For this review, take the finished solid that the model builds, in its own axes (mm). A direction names the side the tool comes from. Round coordinates to 2 decimals unless told otherwise and drop trailing zeros. Write each loop counter-clockwise with the first axis right and the second up, starting at its lowest first coordinate (ties: lowest second). Pieces come first, ordered by that corner, then holes. Notation, with made-up numbers: (-27, 74) -> (13, 74) arc R29 ccw to (13, 100) -> close; hole circle Ø3 at (68, 24). An arc over 180 degrees is marked (long way). Answer in a Markdown table with one row per item. Add a question column.
```python
from build123d import *

# Parameters (mm, degrees)
SKETCH1_R           = 92.5
BOSS_EXTRUDE1_DEPTH = 5
SKETCH2_R           = 72
BOSS_EXTRUDE2_DEPTH = 5
SKETCH3_R           = 67
CUT_EXTRUDE1_DEPTH  = 11
SKETCH4_W           = 140
SKETCH4_H           = 70
BOSS_EXTRUDE3_DEPTH = 5
SKETCH6_W           = 60
SKETCH6_H           = 5
BOSS_EXTRUDE4_DEPTH = 20
FILLET1_R           = 2.5
SKETCH7_W           = 110
SKETCH7_H           = 25
BOSS_EXTRUDE5_DEPTH = 5
SKETCH11_R          = 2
CUT_EXTRUDE4_DEPTH  = 5
SKETCH12_R          = 2.5
CUT_EXTRUDE5_DEPTH  = 5
SKETCH13_R          = 2
CUT_EXTRUDE6_DEPTH  = 5


with BuildPart() as part:
    # Sketch1 → Boss-Extrude1 (new body)
    with BuildSketch(Plane.XY):
        Circle(SKETCH1_R)
    extrude(amount=BOSS_EXTRUDE1_DEPTH)

    # Sketch2 → Boss-Extrude2 (add)
    with BuildSketch(Plane.XY.offset(5)):
        Circle(SKETCH2_R)
    extrude(amount=BOSS_EXTRUDE2_DEPTH)

    # Sketch3 → Cut-Extrude1 (cut, through all)
    with BuildSketch(Plane(origin=(0, 0, 0), x_dir=(-1, 0, 0), z_dir=(0, 0, -1))):
        Circle(SKETCH3_R)
    extrude(amount=-CUT_EXTRUDE1_DEPTH, mode=Mode.SUBTRACT)

    # Sketch4 → Boss-Extrude3 (add)
    with BuildSketch(Plane(origin=(0, 0, 0), x_dir=(-1, 0, 0), z_dir=(0, 0, -1))):
        with Locations((0, -5)):
            Rectangle(SKETCH4_W, SKETCH4_H)
    extrude(amount=-BOSS_EXTRUDE3_DEPTH)

    # Sketch6 → Boss-Extrude4 (add)
    with BuildSketch(Plane.XY.offset(5)):
        with Locations((0, -37.5)):
            Rectangle(SKETCH6_W, SKETCH6_H)
    extrude(amount=BOSS_EXTRUDE4_DEPTH)

    # Fillet1
    fillet1_edges = [part.edges().sort_by_distance(p)[0] for p in [
        (0, -40, 0),
    ]]
    fillet(fillet1_edges, radius=FILLET1_R)

    # Sketch7 → Boss-Extrude5 (add)
    with BuildSketch(Plane(origin=(0, 0, 0), x_dir=(-1, 0, 0), z_dir=(0, 0, -1))):
        with Locations((0, -55)):
            Rectangle(SKETCH7_W, SKETCH7_H)
    extrude(amount=-BOSS_EXTRUDE5_DEPTH)

    # Sketch11 → Cut-Extrude4 (cut)
    with BuildSketch(Plane(origin=(0, 0, 0), x_dir=(-1, 0, 0), z_dir=(0, 0, -1))):
        with Locations((-30, -30)):
            Circle(SKETCH11_R)
        with Locations((-30, 20)):
            Circle(SKETCH11_R)
        with Locations((30, 20)):
            Circle(SKETCH11_R)
        with Locations((30, -30)):
            Circle(SKETCH11_R)
    extrude(amount=-CUT_EXTRUDE4_DEPTH, mode=Mode.SUBTRACT)

    # Sketch12 → Cut-Extrude5 (cut)
    with BuildSketch(Plane(origin=(0, 0, 0), x_dir=(-1, 0, 0), z_dir=(0, 0, -1))):
        with Locations((0, -78.5)):
            Circle(SKETCH12_R)
        with Locations((-78.5, 0)):
            Circle(SKETCH12_R)
        with Locations((0, 78.5)):
            Circle(SKETCH12_R)
        with Locations((78.5, 0)):
            Circle(SKETCH12_R)
    extrude(amount=-CUT_EXTRUDE5_DEPTH, mode=Mode.SUBTRACT)

    # Sketch13 → Cut-Extrude6 (cut)
    with BuildSketch(Plane(origin=(0, -35, 0), x_dir=(1, 0, 0), z_dir=(0, 1, 0))):
        with Locations((-20, -15)):
            Circle(SKETCH13_R)
        with Locations((20, -15)):
            Circle(SKETCH13_R)
    extrude(amount=-CUT_EXTRUDE6_DEPTH, mode=Mode.SUBTRACT)


solid = part.part
```
1. For L1, parallel to Z at x = 20, y = -37; L2, parallel to Y at x = -30, z = 3.7; L3, parallel to Y at x = 29.5, z = 1.5, list the stretches that pass through material, from the lowest coordinate up. Write a range as [from, to].
2. We need section A-A (z = 7.75). Write out the cut boundary in (x, y).
3. The part is to be moulded in two halves that separate along X. For faces 1 (the flat face through (0, -37, 25)), 2 (the cylindrical face through (29.077, -31.774, 2.465)), 3 (the cylindrical face through (49.727, 77.996, 2.465)), say which applies: pulls with the +X half, pulls with the -X half, needs draft (parallel to the pull), parting line crosses it, or undercut.
4. Tool access review of faces 4 (the flat face through (-1, 1, 0)), 5 (the flat face through (1, -40, 14)), 6 (the cylindrical face through (-9.373, 71.387, 7.465)): name each direction out of +Z, -Z, +X, -X, +Y, -Y from which nothing blocks a thin tool from reaching the whole face with its end or side.
5. We need section B-B (x = 0). Count the separate pieces of the cut face and the enclosed holes in it, plus the area to 3 significant figures.
6. We need section C-C (y = 55.5). Write out the cut boundary in (x, z).
7. Clearance check with flat-ended pins moving along their axes: pin 1 Ø2.5 at (x, z) = (-5, 1.5) entering from +Y; pin 2 Ø6.5 at (x, z) = (20, 15) entering from -Y; pin 3 Ø6 at (x, y) = (-78.5, 0) entering from +Z; pin 4 Ø3.5 at (x, y) = (-30, -30) entering from +Z. State where each tip first meets the part, or that it passes through.
8. We need section D-D (x = 78.5). Write out the cut boundary in (y, z).
Response:
| question | item | result |
|---|---|---|
| 1 | L1 | [0, 13], [17, 25] |
| 1 | L2 | [-87.5, -42.5], [-40, -32], [-28, 18], [22, 30], [59.91, 87.5] |
| 1 | L3 | [-87.67, -42.5], [-39.79, -31.94], [-28.06, 18.06], [21.94, 30], [60.16, 87.67] |
| 2 | outline | circle Ø144 at (0, 0); (-30, -40) -> (30, -40) -> (30, -35) -> (-30, -35) -> close; hole circle Ø134 at (0, 0) |
| 3 | face 1 | needs draft |
| 3 | face 2 | undercut |
| 3 | face 3 | parting line crosses it |
| 4 | face 4 | -Z, +X, -X, +Y, -Y |
| 4 | face 5 | +Z, -Z |
| 4 | face 6 | +Z |
| 5 | separate pieces | 5 |
| 5 | enclosed holes | 0 |
| 5 | area | 826 mm2 |
| 6 | outline | (-74, 0) -> (-37.53, 0) -> (-37.53, 10) -> (-45.87, 10) -> (-45.87, 5) -> (-74, 5) -> close; (37.53, 0) -> (74, 0) -> (74, 5) -> (45.87, 5) -> (45.87, 10) -> (37.53, 10) -> close |
| 7 | pin 1 | y = 92.42 |
| 7 | pin 2 | y = -40 |
| 7 | pin 3 | z = 5 |
| 7 | pin 4 | through |
| 8 | outline | (-48.93, 0) -> (-2.5, 0) -> (-2.5, 5) -> (-48.93, 5) -> close; (2.5, 0) -> (48.93, 0) -> (48.93, 5) -> (2.5, 5) -> close |
